Part model, mm, in its own coordinate system. A direction names the side the tool comes from. Round coordinates to 2 decimals unless told otherwise and drop trailing zeros. Loops run counter-clockwise (first coordinate to the right, second up) from the corner with the lowest first, then second, coordinate; pieces in that order, holes last.
from build123d import *

# Parameters (mm, degrees)
F0_W     = 57.15
F0_H     = 44.45
F1_DEPTH = 25.4
F3_DEPTH = 50.8
F5_DEPTH = 12.7


with BuildPart() as f1:
    # F0 (on Front) → F1 (new body)
    with BuildSketch(Plane.XZ):
        with Locations((28.575, 22.225)):
            Rectangle(F0_W, F0_H)
    extrude(amount=-F1_DEPTH)

    # F2 (on face) → F3 (cut)
    with BuildSketch(Plane.XZ):
        with BuildLine():
            ThreePointArc((34.8792097013, 16.7488830228), (37.2675179209, 20.6783904546), (38.1, 25.2007812379))
            ThreePointArc((38.1, 25.2007812379), (33.4601568868, 35.0152537637), (22.930886463, 37.6584486898))
            Line((22.930886463, 37.6584486898), (34.8792097013, 16.7488830228))
        make_face()
        with BuildLine():
            Line((34.8792097013, 16.7488830228), (22.930886463, 37.6584486898))
            ThreePointArc((22.930886463, 37.6584486898), (14.373312095, 18.8998167208), (34.8792097013, 16.7488830228))
        make_face()
    extrude(amount=-F3_DEPTH, mode=Mode.SUBTRACT)

    # F4 (on face) → F5 (cut)
    with BuildSketch(Plane.XZ):
        with BuildLine():
            Line((57.15, 44.45), (19.05, 44.45))
            Line((19.05, 44.45), (22.930886463, 37.6584486898))
            ThreePointArc((22.930886463, 37.6584486898), (33.4601568868, 35.0152537637), (38.1, 25.2007812379))
            ThreePointArc((38.1, 25.2007812379), (37.2675179209, 20.6783904546), (34.8792097013, 16.7488830228))
            Line((34.8792097013, 16.7488830228), (44.45, 0))
            Line((44.45, 0), (57.15, 0))
            Line((57.15, 0), (57.15, 44.45))
        make_face()
    extrude(amount=-F5_DEPTH, mode=Mode.SUBTRACT)


solid = f1.part
1) Drop flat-ended pins along their axis: pin 1 Ø5 at (x, y) = (33.5, 3) entering from -Z; pin 2 Ø4 at (x, z) = (47.5, 22) entering from -Y. Give the stop position or say it passes through.
Values:
pin 1: stops at z = 0
pin 2: stops at y = 12.7
2) Wall check: line 1 along Z through (x, y) = (25.4, 13.75); line 2 along X through (y, z) = (13.5, 14); line 3 along Z through (x, y) = (30, 21.75). Give the ranges that are in metal, low to high.
Values:
line 1: z = 0 to 12.5, 37.9 to 44.45
line 2: x = 0 to 19.41, 31.39 to 57.15
line 3: z = 0 to 13.36, 37.04 to 44.45
3) Slice it at C-C, the plane z = 36.5. Give the cut face in (x, y).
Values:
outline: (0, 0) - (19.6, 0) - (19.6, 25.4) - (0, 25.4) - close; (31.2, 12.7) - (57.15, 12.7) - (57.15, 25.4) - (31.2, 25.4) - close
4) Slice it at B-B, the plane x = 25.4. Give the cut face in (y, z), then the cut area to 3 significant figures.
Values:
outline: (0, 0) - (25.4, 0) - (25.4, 12.5) - (0, 12.5) - close; (12.7, 37.9) - (25.4, 37.9) - (25.4, 44.45) - (12.7, 44.45) - close
area: 401 mm2
5) Slice it at D-D, the plane y = 4.5. Give the cut face in (x, z).
Values:
outline: (0, 0) - (44.45, 0) - (34.88, 16.75) arc R12.7 cw (long way) to (22.93, 37.66) - (19.05, 44.45) - (0, 44.45) - close
6) Tool access for faces 1 (the face through (20.963, 6.261, 41.102)), 2 (the face through (12, 0, 18)): list every direction of +Z, -Z, +X, -X, +Y, -Y with a clear straight run to the whole face (end or side of a thin tool).
Values:
face 1: +Z, +X, -Y
face 2: +Z, -Z, +X, -X, -Y
7) Slice it at A-A, the plane y = 18.25. Give the cut face in (x, z).
Values:
outline: (0, 0) - (57.15, 0) - (57.15, 44.45) - (0, 44.45) - close; hole circle Ø25.4 at (25.4, 25.2)
